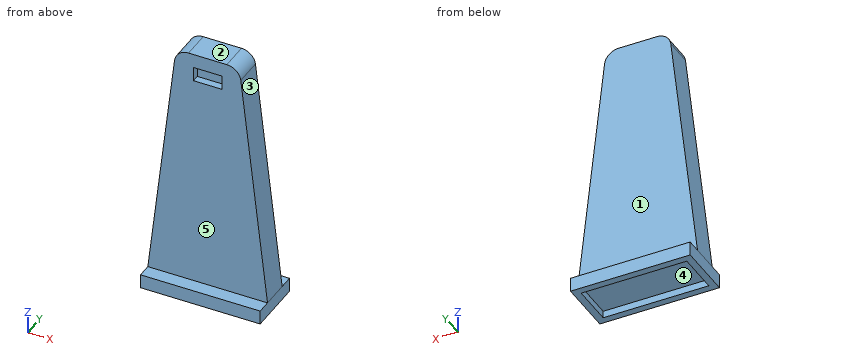
```python
from build123d import *

# Parameters (mm, degrees)
F0_W          = 9
F0_H          = 4
F2_W          = 17
F2_H          = 4
F4_DEPTH      = 2
F5_W          = 17
F5_H          = 2
F6_DEPTH      = 2
F6_DEPTH_BACK = 6
F7_W          = 4.05
F7_H          = 2.05
F8_DEPTH      = 1.05
F9_W          = 14.9999996647
F9_H          = 5.9999996647
F10_DEPTH     = 1
F11_R         = 2


with BuildPart() as f3:
    # F0 (on Top) → F3 section 0
    with BuildSketch(Plane.XY):
        Rectangle(F0_W, F0_H)
    # F2 (on offset) → F3 section 1
    with BuildSketch(Plane.XY.offset(-35)):
        Rectangle(F2_W, F2_H)
    loft()

    # F4 (add): a face of the model
    f4_faces = [f3.faces().sort_by_distance(p)[0] for p in [
        (0, 0, -35),
    ]]
    extrude(f4_faces, amount=F4_DEPTH)

    # F5 (on face) → F6 (join, two sides)
    with BuildSketch(Plane.XZ.offset(2)) as f6_sk:
        with Locations((0, -36)):
            Rectangle(F5_W, F5_H)
    extrude(amount=F6_DEPTH)
    extrude(f6_sk.sketch, amount=-F6_DEPTH_BACK)

    # F7 (on face) → F8 (cut)
    with BuildSketch(Plane.XZ.offset(2)):
        with Locations((0, -3.025)):
            Rectangle(F7_W, F7_H)
    extrude(amount=-F8_DEPTH, mode=Mode.SUBTRACT)

    # F9 (on face) → F10 (cut)
    with BuildSketch(Plane(origin=(0, 0, -37), x_dir=(1, 0, 0), z_dir=(0, 0, -1))):
        Rectangle(F9_W, F9_H)
    extrude(amount=-F10_DEPTH, mode=Mode.SUBTRACT)

    # F11
    f11_edges = [f3.edges().sort_by_distance(p)[0] for p in [
        (-4.5, 0, 0),
        (4.5, 0, 0),
    ]]
    fillet(f11_edges, radius=F11_R)


solid = f3.part
```
Build history of the part. All positions in model axes, mm. Face numbers are marked on the shaded views. A direction names the side the tool comes from. Round coordinates to 2 decimals unless told otherwise and drop trailing zeros. Order: outer loops, then holes, each group sorted by start corner. A loop starts at its lowest first (then second) coordinate and runs counter-clockwise, first axis right, second up. Notation, with made-up numbers: (66.5, 80) - (73.5, 80) arc R21 cw to (73.5, 108) - close; hole circle Ø9 at (62.5, 7.25). An arc over 180 degrees is marked (long way). Use a Markdown table: item, result.
1) Saw through at B-B on x = -1.5. Write the cut outline in (y, z).
Recorded:
| item | result |
|---|---|
| outline | (-4, -37) - (-3, -37) - (-3, -36) - (3, -36) - (3, -37) - (4, -37) - (4, -35) - (2, -35) - (2, 0) - (-2, 0) - (-2, -2) - (-0.95, -2) - (-0.95, -4.05) - (-2, -4.05) - (-2, -35) - (-4, -35) - close |
2) Saw through at D-D on z = -28. Write the cut outline in (x, y).
Recorded:
| item | result |
|---|---|
| outline | (-7.7, -2) - (7.7, -2) - (7.7, 2) - (-7.7, 2) - close |
3) Tool access for the marked faces 1 and 2: list every direction of +Z, -Z, +X, -X, +Y, -Y with a clear straight run to the whole face (end or side of a thin tool).
Recorded:
| item | result |
|---|---|
| face 1 | +Z, +X, -X, +Y |
| face 2 | +Z, +X, -X, +Y, -Y |
4) Pull direction X, two halves, no side cores. Call the marked faces 3, 4 and 5: pulls with the +X half, pulls with the -X half, needs draft (parallel to the pull), parting line crosses it, or undercut.
Recorded:
| item | result |
|---|---|
| face 3 | pulls with the +X half |
| face 4 | undercut |
| face 5 | needs draft |
5) Saw through at A-A on y = -1.5. Write the cut outline in (x, z) (3 decimals), and give its area (3 significant figures).
Recorded:
| item | result |
|---|---|
| outline | (-8.5, -37) - (-7.5, -37) - (-7.5, -36) - (7.5, -36) - (7.5, -37) - (8.5, -37) - (8.5, -35) - (4.703, -1.773) arc R2 ccw to (2.716, 0) - (-2.716, 0) arc R2 ccw to (-4.703, -1.773) - (-8.5, -35) - close; hole (-2.025, -4.05) - (2.025, -4.05) - (2.025, -2) - (-2.025, -2) - close |
| area | 464 mm² |
6) Saw through at C-C on y = 0. Write the cut outline in (x, z).
Recorded:
| item | result |
|---|---|
| outline | (-8.5, -37) - (-7.5, -37) - (-7.5, -36) - (7.5, -36) - (7.5, -37) - (8.5, -37) - (8.5, -35) - (4.7, -1.77) arc R2 ccw to (2.72, 0) - (-2.72, 0) arc R2 ccw to (-4.7, -1.77) - (-8.5, -35) - close |
7) Flat gauge pins, fed straight in: pin 1 Ø8 at (x, z) = (2.5, -4) entering from +Y; pin 2 Ø0.6 at (x, y) = (0.5, 3.5) entering from +Z; pin 3 Ø1.2 at (x, y) = (1, -1.5) entering from -Z. Where does each tip first touch, or does it go through?
Recorded:
| item | result |
|---|---|
| pin 1 | stops at y = 2 |
| pin 2 | stops at z = -35 |
| pin 3 | stops at z = -36 |
8) Wall check: L1, parallel to Y at x = -6, z = -18; L2, parallel to Z at x = -6.75, y = 2.25; L3, parallel to Z at x = 6.25, y = 3.5. Give the ranges that are in metal, low to high.
Recorded:
| item | result |
|---|---|
| L1 | y = -2 to 2 |
| L2 | z = -36 to -35 |
| L3 | z = -37 to -35 |
